Can you work these out from the model? Positions are in its coordinate system, mm. Coordinates: 2 decimals unless noted, no trailing zeros. Order: outer loops, then holes, each group sorted by start corner. A loop starts at its lowest first (then second) coordinate and runs counter-clockwise, first axis right, second up. Notation, with made-up numbers: (-37, -28) -> (-10, -28) arc R27 ccw to (-10, 3) -> close; hole circle Ø6 at (-4, 75). An arc over 180 degrees is marked (long way). Use a Markdown table: item, result. Add a question column.
1. Suppose I cut it at C-C, the plane y = 6.5. List the corners of the cut face in (x, z) for me.
2. Suppose I cut it at D-D, the plane y = -27.25. List the corners of the cut face in (x, z) for me, then the cut area to 3 significant figures.
3. We'd pull the mould along X, two halves only. Please class faces 1 (the cylindrical face through (49.506, -31.686, 2.465)), 2 (the cylindrical face through (-0.209, -45.945, 2.465)), 3 (the flat face through (31.803, -41.352, 2.465)): pulls with the +X half, pulls with the -X half, needs draft (parallel to the pull), parting line crosses it, or undercut.
4. For pin 1 Ø1 at (y, z) = (50.5, 1) entering from +X; pin 2 Ø2 at (y, z) = (-20, 2) entering from +X; pin 3 Ø2 at (y, z) = (-4, 2.5) entering from +X, each with a flat end and sliding along its axis, tell me the tip position at first contact or that it passes through.
5. Suppose I cut it at A-A, the plane x = 0. List the corners of the cut face in (y, z) for me, then the cut area to 3 significant figures.
6. If I drill on line 1 along Y through (x, z) = (0, 1.1); line 2 along Y through (x, z) = (-4, 2.45); line 3 along X through (y, z) = (-26.5, 3.3), over which ranges is the centre line in solid material (lowest first)? Write a range as from..to.
7. Suppose I cut it at B-B, the plane z = 2.8. List the corners of the cut face in (x, y) for me, then the cut area to 3 significant figures.
```python
from build123d import *

# Parameters (mm, degrees)
SKETCH_R   = 35
SKETCH_R_2 = 5
PAD_DEPTH  = 5


with BuildPart() as part:
    # Sketch → Pad (new body)
    with BuildSketch(Plane.XY):
        with BuildLine():
            ThreePointArc((8.339953, 61.67253), (0, 65.5), (-8.339953, 61.67253))
            Line((-8.339953, 61.67253), (-31.16164, 35.136317))
            ThreePointArc((-31.16164, 35.136317), (-39.78947, 22.972461), (-46.009763, 9.418613))
            Line((-46.009763, 9.418613), (-57.579954, -23.613654))
            ThreePointArc((-57.579954, -23.613654), (-56.724664, -32.75), (-49.240001, -38.058876))
            Line((-14.848123, -44.55493), (-49.240001, -38.058876))
            ThreePointArc((-14.848123, -44.55493), (0, -45.944923), (14.848123, -44.55493))
            Line((14.848123, -44.55493), (49.240001, -38.058876))
            ThreePointArc((49.240001, -38.058876), (56.724664, -32.75), (57.579954, -23.613654))
            Line((57.579954, -23.613654), (46.009763, 9.418613))
            ThreePointArc((46.009763, 9.418613), (39.78947, 22.972461), (31.16164, 35.136317))
            Line((8.339953, 61.67253), (31.16164, 35.136317))
        make_face()
        Circle(SKETCH_R, mode=Mode.SUBTRACT)
        with Locations((-47.198385, -27.25)):
            Circle(SKETCH_R_2, mode=Mode.SUBTRACT)
        with Locations((47.198385, -27.25)):
            Circle(SKETCH_R_2, mode=Mode.SUBTRACT)
        with Locations((0, 54.5)):
            Circle(SKETCH_R_2, mode=Mode.SUBTRACT)
    extrude(amount=PAD_DEPTH)


solid = part.part
```
Worked out:
| question | item | result |
|---|---|---|
| 1 | outline | (-47.03, 0) -> (-34.39, 0) -> (-34.39, 5) -> (-47.03, 5) -> close; (34.39, 0) -> (47.03, 0) -> (47.03, 5) -> (34.39, 5) -> close |
| 2 | outline | (-58.2, 0) -> (-52.2, 0) -> (-52.2, 5) -> (-58.2, 5) -> close; (-42.2, 0) -> (-21.96, 0) -> (-21.96, 5) -> (-42.2, 5) -> close; (21.96, 0) -> (42.2, 0) -> (42.2, 5) -> (21.96, 5) -> close; (52.2, 0) -> (58.2, 0) -> (58.2, 5) -> (52.2, 5) -> close |
| 2 | area | 262 mm² |
| 3 | face 1 | undercut |
| 3 | face 2 | parting line crosses it |
| 3 | face 3 | pulls with the +X half |
| 4 | pin 1 | stops at x = 18.38 |
| 4 | pin 2 | stops at x = 56.66 |
| 4 | pin 3 | stops at x = 51.06 |
| 5 | outline | (-45.94, 0) -> (-35, 0) -> (-35, 5) -> (-45.94, 5) -> close; (35, 0) -> (49.5, 0) -> (49.5, 5) -> (35, 5) -> close; (59.5, 0) -> (65.5, 0) -> (65.5, 5) -> (59.5, 5) -> close |
| 5 | area | 157 mm² |
| 6 | line 1 | y = -45.94..-35, 35..49.5, 59.5..65.5 |
| 6 | line 2 | y = -45.84..-34.77, 34.77..51.5, 57.5..64.75 |
| 6 | line 3 | x = -58.17..-52.14, -42.25..-22.86, 22.86..42.25, 52.14..58.17 |
| 7 | outline | (-57.58, -23.61) arc R11 ccw to (-49.24, -38.06) -> (-14.85, -44.55) arc R80 ccw to (14.85, -44.55) -> (49.24, -38.06) arc R11 ccw to (57.58, -23.61) -> (46.01, 9.42) arc R80 ccw to (31.16, 35.14) -> (8.34, 61.67) arc R11 ccw to (-8.34, 61.67) -> (-31.16, 35.14) arc R80 ccw to (-46.01, 9.42) -> close; hole circle Ø10 at (-47.2, -27.25); hole circle Ø70 at (0, 0); hole circle Ø10 at (0, 54.5); hole circle Ø10 at (47.2, -27.25) |
| 7 | area | 4,550 mm² |
